from build123d import *

# Parameters (mm, degrees)
SKETCH1_R                = 38.1
CENTERHUB_DEPTH          = 20.6375
RIB_DEPTH                = 3.175
LIGHTENING_HOLE_DEPTH    = 253.292660231
FILLET1_R                = 6.35
CIRPATTERN1_COUNT        = 6
FILLET1_OF_CIRPATTERN1_R = 6.35
THRU_HOLE_DEPTH          = 253.292660231
THRU_HOLE_DEPTH_BACK     = 253.292660231
SKETCH5_R                = 19.05


with BuildPart() as part:
    # Sketch1 → CenterHub (new, symmetric)
    with BuildSketch(Plane.XY):
        Circle(SKETCH1_R)
    extrude(amount=CENTERHUB_DEPTH, both=True)

    # Sketch2 → Rim and Web (revolve)
    with BuildSketch(Plane(origin=(0, 0, 0), x_dir=(0, 0, -1), z_dir=(1, 0, 0)), mode=Mode.PRIVATE) as rim_and_web_sk:
        Polygon((-6.35, 0), (6.35, 0), (6.35, 165.1), (19.05, 165.1), (19.05, 177.8), (-19.05, 177.8), (-19.05, 165.1), (-6.35, 165.1), align=None)
    revolve(rim_and_web_sk.sketch.rotate(Axis((0, 0, 0), (0, 0, -1)), 90), axis=Axis((0, 0, 0), (0, 0, -1)))

    # Sketch3 → Rib (add, symmetric)
    with BuildSketch(Plane(origin=(0, 0, 0), x_dir=(1, 0, 0), z_dir=(0, 1, 0))):
        Polygon((0, -19.05), (132.747036773, -19.05), (167.64, -6.35), (167.64, 6.35), (132.747036773, 19.05), (0, 19.05), align=None)
    rib = extrude(amount=RIB_DEPTH, both=True)

    # Sketch4 → Lightening hole (cut, symmetric)
    with BuildSketch(Plane.XY):
        with BuildLine():
            Line((92.100127656, -121.422100483), (43.438552305, -37.1377796))
            ThreePointArc((43.438552305, -37.1377796), (49.493351826, -28.575), (53.881536726, -19.05))
            Line((53.881536726, -19.05), (151.204687427, -19.05))
            ThreePointArc((151.204687427, -19.05), (131.982271537, -76.2), (92.100127656, -121.422100483))
        make_face()
    lightening_hole = extrude(amount=LIGHTENING_HOLE_DEPTH, both=True, mode=Mode.SUBTRACT)

    # Fillet1
    fillet1_edges = [part.edges().sort_by_distance(p)[0] for p in [
        (151.204687427, -19.05, 0),
        (92.100127656, -121.422100483, 0),
        (43.438552305, -37.1377796, 0),
        (53.881536726, -19.05, 0),
    ]]
    fillet(fillet1_edges, radius=FILLET1_R)

    # CirPattern1: Rib, Lightening hole ×6 about axis
    cirpattern1_axis = Axis((0, 0, 0), (0, 0, 1))
    add([rib.rotate(cirpattern1_axis, i * 360 / CIRPATTERN1_COUNT) for i in range(1, CIRPATTERN1_COUNT)])
    add([lightening_hole.rotate(cirpattern1_axis, i * 360 / CIRPATTERN1_COUNT) for i in range(1, CIRPATTERN1_COUNT)], mode=Mode.SUBTRACT)

    # Fillet1 of CirPattern1
    fillet1_of_cirpattern1_edges = [part.edges().sort_by_distance(p)[0] for p in [
        (92.100127656, 121.422100483, 0),
        (151.204687427, 19.05, 0),
        (53.881536726, 19.05, 0),
        (43.438552305, 37.1377796, 0),
        (-59.104559772, 140.472100483, 0),
        (59.104559772, 140.472100483, 0),
        (10.442984421, 56.1877796, 0),
        (-10.442984421, 56.1877796, 0),
        (-151.204687427, 19.05, 0),
        (-92.100127656, 121.422100483, 0),
        (-43.438552305, 37.1377796, 0),
        (-53.881536726, 19.05, 0),
        (-92.100127656, -121.422100483, 0),
        (-151.204687427, -19.05, 0),
        (-53.881536726, -19.05, 0),
        (-43.438552305, -37.1377796, 0),
        (59.104559772, -140.472100483, 0),
        (-59.104559772, -140.472100483, 0),
        (-10.442984421, -56.1877796, 0),
        (10.442984421, -56.1877796, 0),
    ]]
    fillet(fillet1_of_cirpattern1_edges, radius=FILLET1_OF_CIRPATTERN1_R)

    # Sketch5 → Thru hole (cut, two sides: drawn at the far end of the back side and taken through both)
    with BuildSketch(Plane.XY.offset(-THRU_HOLE_DEPTH_BACK)):
        Circle(SKETCH5_R)
    extrude(amount=THRU_HOLE_DEPTH + THRU_HOLE_DEPTH_BACK, mode=Mode.SUBTRACT)


solid = part.part
Design review of the part built by this model. Coordinates are the model's own, in mm. A direction names the side the tool comes from. Coordinates: 2 decimals unless noted, no trailing zeros. Loops run counter-clockwise (first coordinate to the right, second up) from the corner with the lowest first, then second, coordinate; pieces in that order, holes last. Notation, with made-up numbers: (30.5, -37) - (35.5, -37) arc R18 cw to (35.5, -12) - close; hole circle Ø6 at (-29.75, -16). An arc over 180 degrees is marked (long way). Use CSV: the item, a comma, the result in double quotes. Start each with the question number.
1. Add section A-A on x = 0. Count the separate pieces of the cut face and the enclosed holes in it, plus the area to 3 significant figures.
2. For faces 4 (the flat face through (36, -100, -6.35)), 5 (the flat face through (7.9, 17.5, -20.638)), 6 (the flat face through (101, 3.175, 13)), 7 (the flat face through (-67.3, 78.47, 0.09)), list the 3-axis set-ups (+Z, -Z, +X, -X, +Y, -Y) from which the entire face can be reached by the end or side of a thin tool; tool diameter is ignored.
3. Mouldability with a two-part tool opening along X and no side actions: class faces 1 (the cylindrical face through (-55.855, -139.501, 0.089)), 2 (the flat face through (-34.308, -97.523, 0.089)), 3 (the flat face through (52, 157, 19.05)) as released by +X, released by -X, zero draft, split by the parting line, or undercut.
4. Add section B-B on z = 13.5. Give the boundary of the cut face in (x, y) (3 decimals).
5. To check wall thickness, follow probe 1 along Y at (x, z) = (0, -14.5); probe 2 along Y at (x, z) = (-92.5, 16.5) (3 decimals); probe 3 along Y at (x, z) = (-119, -15) (3 decimals). State the ranges of each line that lie inside material, in increasing order.
6. Add section C-C on x = -108. Give the boundary of the cut face in (y, z) (3 decimals).
7. Clearance check with flat-ended pins moving along their axes: pin 1 (16 mm diameter, centred on x = -55, y = -62.5, fed in from -Z); pin 2 (14 mm diameter, centred on x = 83.5, z = 14, fed in from -Y); pin 3 (14 mm diameter, centred on x = 85, z = -3, fed in from -Y). State where each tip first meets the part, or that it passes through.
Resolved:
1,separate pieces,"4"
1,enclosed holes,"0"
1,area,"3,350 mm2"
2,face 4,"-Z"
2,face 5,"-Z, +X, -X, +Y, -Y"
2,face 6,"+Z"
2,face 7,"+Z, -Z"
3,face 1,"undercut"
3,face 2,"undercut"
3,face 3,"zero draft"
4,outline,"circle Ø355.6 at (0, 0); (-147.996, -3.175) - (-37.967, -3.175) arc R38.1 ccw to (-21.733, -31.293) - (-76.747, -126.58) - (-71.248, -129.755) - (-16.234, -34.468) arc R38.1 ccw to (16.234, -34.468) - (71.248, -129.755) - (76.747, -126.58) - (21.733, -31.293) arc R38.1 ccw to (37.967, -3.175) - (147.996, -3.175) - (147.996, 3.175) - (37.967, 3.175) arc R38.1 ccw to (21.733, 31.293) - (76.747, 126.58) - (71.248, 129.755) - (16.234, 34.468) arc R38.1 ccw to (-16.234, 34.468) - (-71.248, 129.755) - (-76.747, 126.58) - (-21.733, 31.293) arc R38.1 ccw to (-37.967, 3.175) - (-147.996, 3.175) - close; hole circle Ø330.2 at (0, 0); hole circle Ø38.1 at (0, 0)"
5,probe 1,"-177.8 to -165.1, -38.1 to -19.05, 19.05 to 38.1, 165.1 to 177.8"
5,probe 2,"-151.844 to -136.754, -3.175 to 3.175, 136.754 to 151.844"
5,probe 3,"-132.105 to -114.442, -3.175 to 3.175, 114.442 to 132.105"
6,outline,"(-141.24, -19.05) - (-124.876, -19.05) - (-124.876, -6.35) - (-107.526, -6.35) - (-107.526, 6.35) - (-124.876, 6.35) - (-124.876, 19.05) - (-141.24, 19.05) - close; (-19.05, -6.35) - (-3.175, -6.35) - (-3.175, -19.05) - (3.175, -19.05) - (3.175, -6.35) - (19.05, -6.35) - (19.05, 6.35) - (3.175, 6.35) - (3.175, 19.05) - (-3.175, 19.05) - (-3.175, 6.35) - (-19.05, 6.35) - close; (107.526, -6.35) - (124.876, -6.35) - (124.876, -19.05) - (141.24, -19.05) - (141.24, 19.05) - (124.876, 19.05) - (124.876, 6.35) - (107.526, 6.35) - close"
7,pin 1,"z = -6.35"
7,pin 2,"y = -160.5"
7,pin 3,"y = -159.78"
